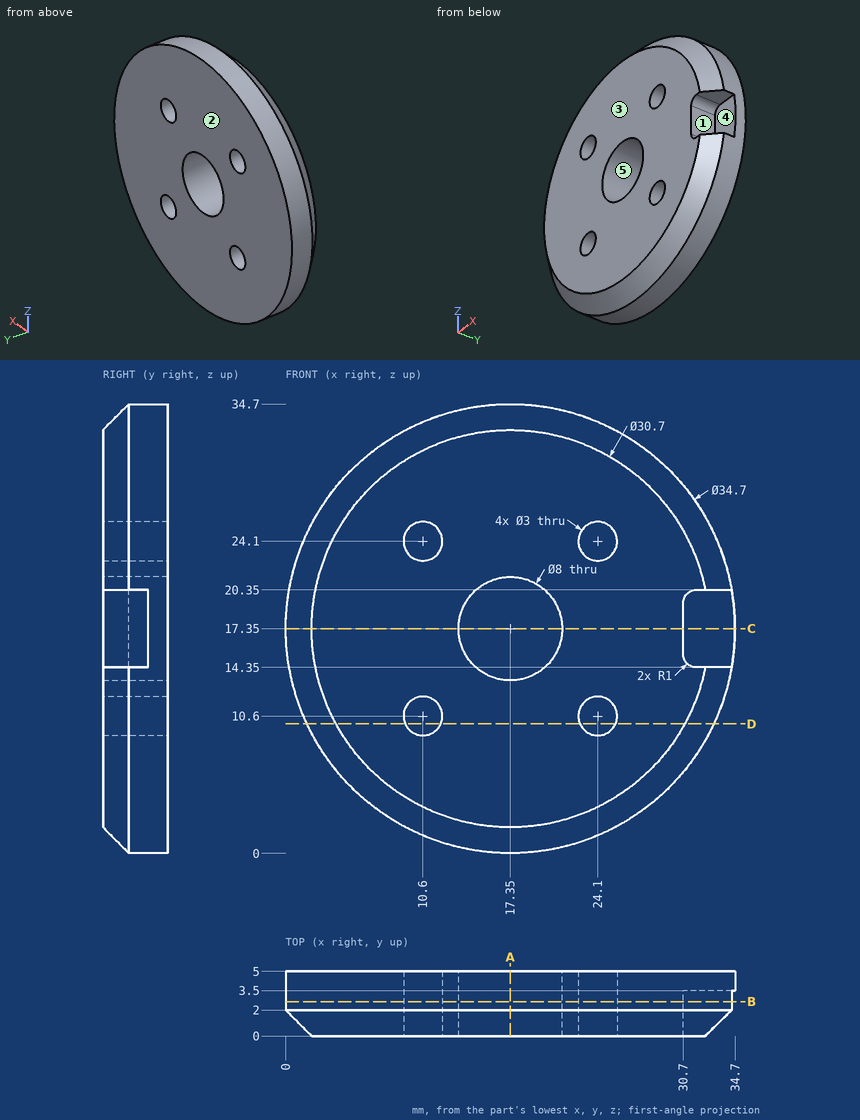
Job drawing, mm, ordinate dimensions from the low corner. One solid piece. A direction names the side the tool comes from. Give positions to 0.01 mm unless a question says otherwise; leave off trailing zeros. Order: outer loops, then holes, each group sorted by start corner. A loop starts at its lowest first (then second) coordinate and runs counter-clockwise, first axis right, second up. Notation, with made-up numbers: (37, -12) - (50, -12) arc R19 cw to (50, 24) - close; hole circle Ø10 at (3.5, 3). An arc over 180 degrees is marked (long way). Return JSON: item names as keys, results as strings.
1) Pull direction Y, two halves, no side cores. Call the marked faces 1, 2 and 3: pulls with the +Y half, pulls with the -Y half, needs draft (parallel to the pull), parting line crosses it, or undercut.
Geometry says:
{"face 1": "needs draft", "face 2": "pulls with the +Y half", "face 3": "pulls with the -Y half"}
2) Cut at A-A, the plane x = 17.35. Give the cut face in (y, z), plus the area to 4 significant figures.
Geometry says:
{"outline": "(0, 2) - (2, 0) - (5, 0) - (5, 13.35) - (0, 13.35) - close; (0, 21.35) - (5, 21.35) - (5, 34.7) - (2, 34.7) - (0, 32.7) - close", "area": "129.5 mm²"}
3) Probe line 1 (X direction, y = 4.8, z = 17.5); line 2 (X direction, y = 3.8, z = 24.1); line 3 (X direction, y = 2.65, z = 24). List the from-to ranges inside material, lowest first. Write a range as from..to.
Geometry says:
{"line 1": "0..13.35, 21.35..34.7", "line 2": "1.37..9.1, 12.1..22.6, 25.6..33.33", "line 3": "1.33..9.1, 12.1..22.6, 25.6..33.37"}
4) Cut at D-D, the plane z = 10. Count the separate pieces of the cut face and the enclosed holes in it, plus the area to 3 significant figures.
Geometry says:
{"separate pieces": "3", "enclosed holes": "0", "area": "125 mm²"}
5) Cut at B-B, the plane y = 2.65. Give the cut face in (x, z), plus the area to 3 significant figures.
Geometry says:
{"outline": "(30.7, 15.35) - (30.7, 19.35) arc R1 cw to (31.7, 20.35) - (34.44, 20.35) arc R17.35 ccw (long way) to (34.44, 14.35) - (31.7, 14.35) arc R1 cw to start; hole circle Ø3 at (10.6, 10.6); hole circle Ø3 at (10.6, 24.1); hole circle Ø8 at (17.35, 17.35); hole circle Ø3 at (24.1, 10.6); hole circle Ø3 at (24.1, 24.1)", "area": "844 mm²"}
6) 3-axis set-ups, long thin cutter, end or side, ignore diameter. For the marked faces 4 and 5: which of +Z, -Z, +X, -X, +Y, -Y reach the whole face in a straight line?
Geometry says:
{"face 4": "+X, -Y", "face 5": "+Y, -Y"}
7) Cut at C-C, the plane z = 17.35. Give the cut face in (x, y).
Geometry says:
{"outline": "(0, 2) - (2, 0) - (13.35, 0) - (13.35, 5) - (0, 5) - close; (21.35, 0) - (30.7, 0) - (30.7, 3.5) - (34.7, 3.5) - (34.7, 5) - (21.35, 5) - close"}
8) Flat gauge pins, fed straight in: P1, Ø1, axis at x = 30.5, y = 3, coming from the +Z side; P2, Ø3, axis at x = 32.5, y = 2.5, coming from the -Z side; P3, Ø10.5, axis at x = 17.35, z = 17.35, coming from the +Y side; P4, Ø1.5, axis at y = 2, z = 26.5, coming from the -X side. Where does each tip first touch, or does it go through?
Geometry says:
{"P1": "z = 29.22", "P2": "z = 6.64", "P3": "y = 5", "P4": "x = 2.17"}
